Verification items for the finished model (mm, model axes). A direction names the side the tool comes from. Give positions to 0.01 mm unless a question says otherwise; leave off trailing zeros. Loops run counter-clockwise (first coordinate to the right, second up) from the corner with the lowest first, then second, coordinate; pieces in that order, holes last. Notation, with made-up numbers: (17, 61.5) - (44, 61.5) arc R25 ccw to (44, 96.5) - close; hole circle Ø7 at (42.5, -7). An arc over 180 degrees is marked (long way). One line per question, with ' | ' between items. Start each with the question number.
1. Tool access check on faces 4 (the face through (-4, -5, 2.2)), 5 (the face through (-4, -4, 2.6)), 6 (the face through (4, 4, 2.6)), 7 (the face through (-4.75, -1, 1)). Record the directions out of +Z, -Z, +X, -X, +Y, -Y that give a thin tool (end or side, any length) a straight path to the whole face; none if there is none.
2. Section check D-D, the plane y = -0.25. Enter the section's corners in (x, z), then the cut area to 3 significant figures.
3. Section check C-C, the plane y = 3.65. Enter the section's corners in (x, z), then the cut area to 3 significant figures.
4. Section check B-B, the plane x = -3.8. Enter the section's corners in (y, z).
5. Section check A-A, the plane z = 3.35. Enter the section's corners in (x, y).
6. Thickness scan on line 1 along Z through (x, y) = (-2.25, 2.75); line 2 along Z through (x, y) = (-4, -4); line 3 along Y through (x, z) = (0.75, 3.55). Record the ranges inside material, lowest first. Write a range as from..to.
7. Mould release check, pull along Y, two halves, no side actions. Record for faces 1 (the face through (3, 3, 2.2)), 2 (the face through (0, -6.25, 1)), 3 (the face through (0, -1, 0)): +Y half, -Y half, draft (parallel to the pull), parting line (faces both ways), or undercut.
8. Depth check by flat-ended pin: pin 1 Ø1.9 at (x, y) = (3.5, 4) entering from +Z; pin 2 Ø1 at (x, y) = (0.5, 0) entering from +Z; pin 3 Ø0.9 at (x, z) = (0, 3.5) entering from +Y. Enter the tip coordinate at first touch or a pass-through.
from build123d import *

# Parameters (mm, degrees)
SKETCH_W     = 9.5
SKETCH_H     = 11.1
PAD_DEPTH    = 3
POCKET_DEPTH = 0.8
SKETCH002_R  = 0.8
PAD001_DEPTH = 0.4
SKETCH003_R  = 0.8
PAD002_DEPTH = 0.4
FILLET_R     = 0.2
FILLET001_R  = 0.5
PAD003_DEPTH = 0.8


with BuildPart() as part:
    # Sketch → Pad (new body)
    with BuildSketch(Plane.XY):
        with Locations((0, -0.7)):
            Rectangle(SKETCH_W, SKETCH_H)
    extrude(amount=PAD_DEPTH)

    # Sketch001 (on Face6 of Pad) → Pocket (cut)
    with BuildSketch(Plane.XY.offset(3)):
        with BuildLine():
            Line((-3.42, -2.28), (-4.75, -2.28))
            Line((-4.75, -2.28), (-4.75, -6.25))
            Line((-4.75, -6.25), (-2.42, -6.25))
            Line((-2.42, -6.25), (-2.42, -3.28))
            ThreePointArc((-2.42, -3.28), (-2.712893, -2.572893), (-3.42, -2.28))
        make_face()
        with BuildLine():
            Line((4.75, 2.28), (4.75, 4.85))
            Line((4.75, 4.85), (2.42, 4.85))
            Line((2.42, 4.85), (2.42, 3.28))
            ThreePointArc((2.42, 3.28), (2.712893, 2.572893), (3.42, 2.28))
            Line((4.75, 2.28), (3.42, 2.28))
        make_face()
    extrude(amount=-POCKET_DEPTH, mode=Mode.SUBTRACT)

    # Sketch002 (on Face4 of Pocket) → Pad001 (join)
    with BuildSketch(Plane.XY.offset(2.2)):
        with Locations((-3.8, -3.65)):
            Circle(SKETCH002_R)
    extrude(amount=PAD001_DEPTH)

    # Sketch003 (on Face4 of Pad001) → Pad002 (join)
    with BuildSketch(Plane.XY.offset(2.2)):
        with Locations((3.8, 3.65)):
            Circle(SKETCH003_R)
    extrude(amount=PAD002_DEPTH)

    # Fillet
    fillet_edges = [part.edges().sort_by_distance(p)[0] for p in [
        (-4.6, -3.65, 2.6),
        (3, 3.65, 2.6),
    ]]
    fillet(fillet_edges, radius=FILLET_R)

    # Fillet001
    fillet001_edges = [part.edges().sort_by_distance(p)[0] for p in [
        (4.75, 4.85, 1.1),
        (-4.75, 4.85, 1.5),
        (-4.75, -6.25, 1.1),
        (4.75, -6.25, 1.5),
    ]]
    fillet(fillet001_edges, radius=FILLET001_R)

    # Sketch005 (on Face11 of Fillet001) → Pad003 (join)
    with BuildSketch(Plane.XY.offset(3)):
        with BuildLine():
            Line((-0.8, -5.45), (0.8, -5.45))
            ThreePointArc((1, -5.65), (0.941421, -5.508579), (0.8, -5.45))
            Line((1, -5.65), (1, -6.05))
            ThreePointArc((0.8, -6.25), (0.941421, -6.191421), (1, -6.05))
            Line((0.8, -6.25), (-0.8, -6.25))
            ThreePointArc((-1, -6.05), (-0.941421, -6.191421), (-0.8, -6.25))
            Line((-1, -6.05), (-1, -5.65))
            ThreePointArc((-0.8, -5.45), (-0.941421, -5.508579), (-1, -5.65))
        make_face()
    extrude(amount=PAD003_DEPTH)


solid = part.part
Results list:
1) face 4: +Z | face 5: +Z, -X, -Y | face 6: +Z, +X, +Y | face 7: +Z, -Z, -X, +Y, -Y
2) outline: (-4.75, 0) - (4.75, 0) - (4.75, 3) - (-4.75, 3) - close | area: 28.5 mm²
3) outline: (-4.75, 0) - (4.75, 0) - (4.75, 2.2) - (4.6, 2.2) - (4.6, 2.4) arc R0.2 ccw to (4.4, 2.6) - (3.2, 2.6) arc R0.2 ccw to (3, 2.4) - (3, 2.2) - (2.42, 2.2) - (2.42, 3) - (-4.75, 3) - close | area: 27.3 mm²
4) outline: (-6.25, 0) - (4.85, 0) - (4.85, 3) - (-2.28, 3) - (-2.28, 2.2) - (-2.85, 2.2) - (-2.85, 2.4) arc R0.2 ccw to (-3.05, 2.6) - (-4.25, 2.6) arc R0.2 ccw to (-4.45, 2.4) - (-4.45, 2.2) - (-6.25, 2.2) - close
5) outline: (-1, -6.05) arc R0.2 ccw to (-0.8, -6.25) - (0.8, -6.25) arc R0.2 ccw to (1, -6.05) - (1, -5.65) arc R0.2 ccw to (0.8, -5.45) - (-0.8, -5.45) arc R0.2 ccw to (-1, -5.65) - close
6) line 1: 0..3 | line 2: 0..2.6 | line 3: -6.25..-5.45
7) face 1: undercut | face 2: -Y half | face 3: draft
8) pin 1: z = 2.6 | pin 2: z = 3 | pin 3: y = -5.45
